Geometry check sheet. Reference: the model listing, model coordinates, mm. Face numbers are marked on the shaded views. Round coordinates to 2 decimals unless told otherwise and drop trailing zeros. Write each loop counter-clockwise with the first axis right and the second up, starting at its lowest first coordinate (ties: lowest second). Pieces come first, ordered by that corner, then holes. Notation, with made-up numbers: (88, 21) -> (100, 21) arc R22 cw to (100, 51) -> close; hole circle Ø5 at (-33.5, -16). An arc over 180 degrees is marked (long way). Use a Markdown table: item, result.
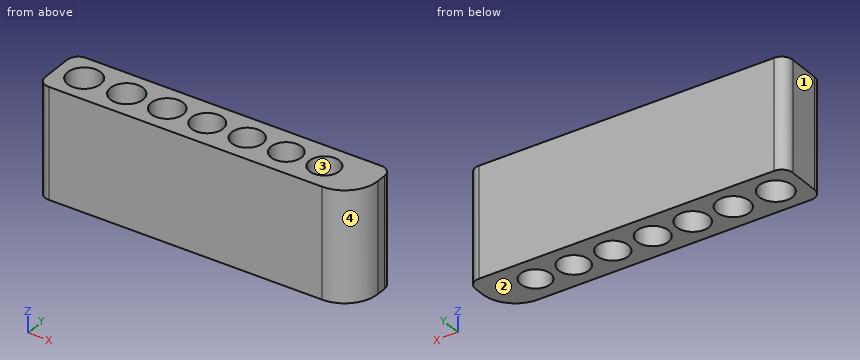
```python
from build123d import *

# Parameters (mm, degrees)
F0_R     = 1.5
F0_R_2   = 1.475
F0_R_3   = 1.45
F0_R_4   = 1.425
F0_R_5   = 1.4
F0_R_6   = 1.375
F0_R_7   = 1.35
F1_DEPTH = 10


with BuildPart() as f1:
    # F0 (on Top) → F1 (new body)
    with BuildSketch(Plane.XY):
        with BuildLine():
            Line((25.263883, 2.41127), (-1.497099, 2.41127))
            ThreePointArc((-1.497099, 2.41127), (-2.204206, 2.118377), (-2.497099, 1.41127))
            Line((-2.497099, 1.41127), (-2.497099, -1.495804))
            ThreePointArc((-2.497099, -1.495804), (-2.204206, -2.202911), (-1.497099, -2.495804))
            Line((-1.497099, -2.495804), (23.263883, -2.495804))
            ThreePointArc((23.263883, -2.495804), (25.385203, -1.617124), (26.263883, 0.504196))
            Line((26.263883, 0.504196), (26.263883, 1.41127))
            ThreePointArc((26.263883, 1.41127), (25.97099, 2.118377), (25.263883, 2.41127))
        make_face()
        Circle(F0_R, mode=Mode.SUBTRACT)
        with Locations((3.857963, 0)):
            Circle(F0_R_2, mode=Mode.SUBTRACT)
        with Locations((7.531565, 0)):
            Circle(F0_R_3, mode=Mode.SUBTRACT)
        with Locations((11.151538, 0)):
            Circle(F0_R_4, mode=Mode.SUBTRACT)
        with Locations((14.771511, 0)):
            Circle(F0_R_5, mode=Mode.SUBTRACT)
        with Locations((18.311039, 0)):
            Circle(F0_R_6, mode=Mode.SUBTRACT)
        with Locations((21.770123, 0)):
            Circle(F0_R_7, mode=Mode.SUBTRACT)
    extrude(amount=F1_DEPTH)


solid = f1.part
```
(1) Section check A-A on z = 8. Record the cut outline in (x, y) (3 decimals), plus the area to 3 significant figures.
A:
| item | result |
|---|---|
| outline | (-2.497, -1.496) arc R1 ccw to (-1.497, -2.496) -> (23.264, -2.496) arc R3 ccw to (26.264, 0.504) -> (26.264, 1.411) arc R1 ccw to (25.264, 2.411) -> (-1.497, 2.411) arc R1 ccw to (-2.497, 1.411) -> close; hole circle Ø3 at (0, 0); hole circle Ø2.95 at (3.858, 0); hole circle Ø2.9 at (7.532, 0); hole circle Ø2.85 at (11.152, 0); hole circle Ø2.8 at (14.772, 0); hole circle Ø2.75 at (18.311, 0); hole circle Ø2.7 at (21.77, 0) |
| area | 93.8 mm2 |
(2) Gauge pin test, flat end, axial feed: pin 1 Ø1.8 at (x, y) = (3.86, 0) entering from -Z. Record the tip position at first contact, or that the pin passes through.
A:
| item | result |
|---|---|
| pin 1 | passes through |
(3) Section check B-B on x = 0. Record the cut outline in (y, z), plus the area to 3 significant figures.
A:
| item | result |
|---|---|
| outline | (-2.5, 0) -> (-1.5, 0) -> (-1.5, 10) -> (-2.5, 10) -> close; (1.5, 0) -> (2.41, 0) -> (2.41, 10) -> (1.5, 10) -> close |
| area | 19.1 mm2 |
(4) Section check D-D on x = 14.25. Record the cut outline in (y, z), plus the area to 3 significant figures.
A:
| item | result |
|---|---|
| outline | (-2.5, 0) -> (-1.3, 0) -> (-1.3, 10) -> (-2.5, 10) -> close; (1.3, 0) -> (2.41, 0) -> (2.41, 10) -> (1.3, 10) -> close |
| area | 23.1 mm2 |
(5) Section check C-C on y = -0.9. State how many separate pieces and enclosed holes the cut face has, plus the area to 3 significant figures.
A:
| item | result |
|---|---|
| separate pieces | 8 |
| enclosed holes | 0 |
| area | 130 mm2 |
(6) Release check for a two-part mould opening along X. For the marked faces 1, 2, 3 and 4 record: +X half, -X half, draft (parallel to the pull), parting line (faces both ways), or undercut.
A:
| item | result |
|---|---|
| face 1 | -X half |
| face 2 | draft |
| face 3 | undercut |
| face 4 | +X half |
(7) Thickness scan on line 1 (Y direction, x = 0.25, z = 8.25); line 2 (Y direction, x = 3.5, z = 5); line 3 (X direction, y = 2.05, z = 5.5). Record the ranges inside material, lowest first.
A:
| item | result |
|---|---|
| line 1 | y = -2.5 to -1.48, 1.48 to 2.41 |
| line 2 | y = -2.5 to -1.43, 1.43 to 2.41 |
| line 3 | x = -2.27 to 26.03 |
